Answer from the drawing. Dimensions are ordinates in mm from the lowest x, y and z of the part. Round coordinates to 2 decimals unless told otherwise and drop trailing zeros. Order: outer loops, then holes, each group sorted by start corner. A loop starts at its lowest first (then second) coordinate and runs counter-clockwise, first axis right, second up.
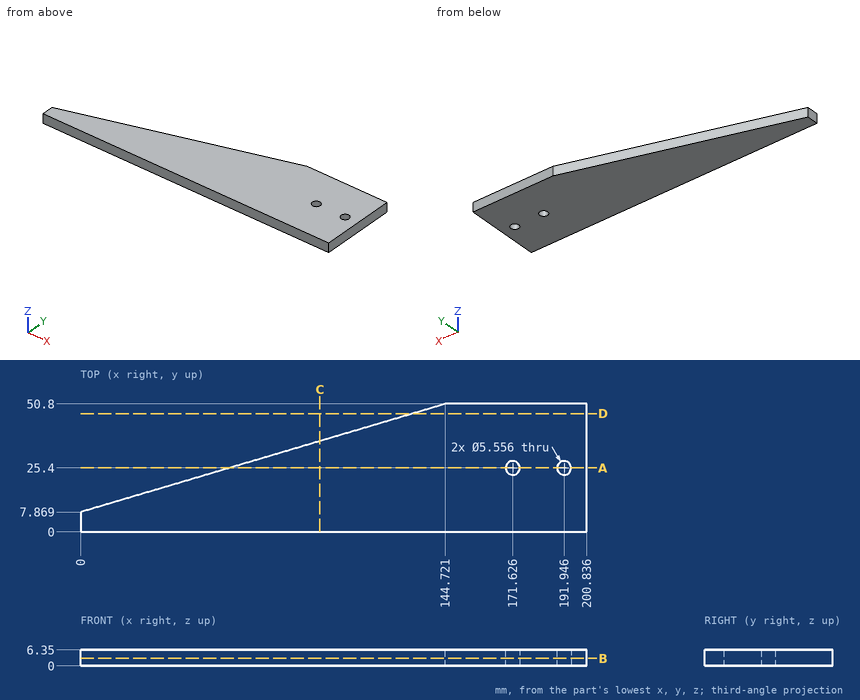
Q1. A cutting plane is placed at A-A, the plane y = 25.4. Give the number of separate pieces and of enclosed holes in the cut face.
Outcome:
separate pieces: 3
enclosed holes: 0
Q2. A cutting plane is placed at D-D, the plane y = 47. Give the vertices of the cut face in (x, z).
Outcome:
outline: (131.91, 0) - (200.84, 0) - (200.84, 6.35) - (131.91, 6.35) - close
Q3. A cutting plane is placed at B-B, the plane z = 3. Give the vertices of the cut face in (x, y) (1 decimal).
Outcome:
outline: (0, 0) - (200.8, 0) - (200.8, 50.8) - (144.7, 50.8) - (0, 7.9) - close; hole circle Ø5.6 at (171.6, 25.4); hole circle Ø5.6 at (191.9, 25.4)
Q4. Straight lines are drawn through the part: probe 1 along Y at (x, z) = (126, 5.25); probe 2 along Y at (x, z) = (54.5, 1.5). For each, find the intervals that lie inside material, in ascending order.
Outcome:
probe 1: y = 0 to 45.25
probe 2: y = 0 to 24.04
Q5. A cutting plane is placed at C-C, the plane x = 95. Give the vertices of the cut face in (y, z).
Outcome:
outline: (0, 0) - (36.05, 0) - (36.05, 6.35) - (0, 6.35) - close
